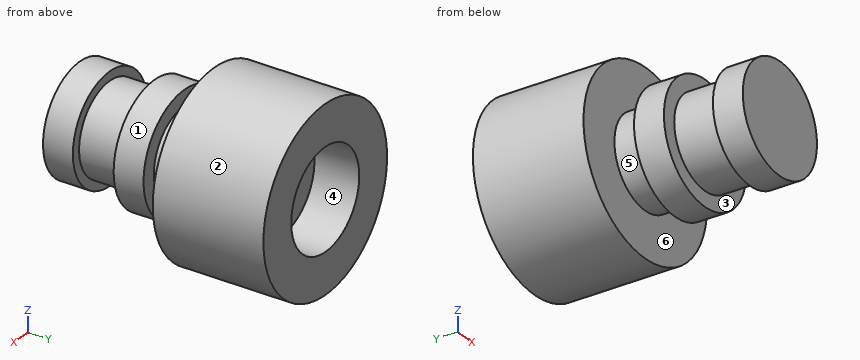
```python
from build123d import *

# Parameters (mm, degrees)
SKETCH1_R           = 3
BOSS_EXTRUDE1_DEPTH = 3.7
SKETCH1_3_R         = 1.6
BOSS_EXTRUDE2_DEPTH = 1
SKETCH5_R           = 1.5
BOSS_EXTRUDE3_DEPTH = 1
SKETCH6_R           = 2
BOSS_EXTRUDE4_DEPTH = 1
SKETCH8_R           = 1.5
BOSS_EXTRUDE5_DEPTH = 2.5
SKETCH10_R          = 1.8
BOSS_EXTRUDE6_DEPTH = 1
SKETCH12_R          = 1.65
CUT_EXTRUDE1_DEPTH  = 1.5


with BuildPart() as part:
    # Sketch1 → Boss-Extrude1 (new body)
    with BuildSketch(Plane(origin=(0, 0, 0), x_dir=(1, 0, 0), z_dir=(0, 1, 0))):
        with Locations((-0.522013312, 0.511138034)):
            Circle(SKETCH1_R)
    extrude(amount=BOSS_EXTRUDE1_DEPTH)

    # Sketch1<3> → Boss-Extrude2 (add)
    with BuildSketch(Plane(origin=(0, 0, 0), x_dir=(1, 0, 0), z_dir=(0, 1, 0))):
        with Locations((-0.522013312, 0.511138034)):
            Circle(SKETCH1_3_R)
    extrude(amount=BOSS_EXTRUDE2_DEPTH)

    # Sketch5 → Boss-Extrude3 (add)
    with BuildSketch(Plane.XZ):
        with Locations((-0.522013312, -0.511138034)):
            Circle(SKETCH5_R)
    extrude(amount=BOSS_EXTRUDE3_DEPTH)

    # Sketch6 → Boss-Extrude4 (add)
    with BuildSketch(Plane.XZ.offset(1)):
        with Locations((-0.522013312, -0.511138034)):
            Circle(SKETCH6_R)
    extrude(amount=BOSS_EXTRUDE4_DEPTH)

    # Sketch8 → Boss-Extrude5 (add)
    with BuildSketch(Plane(origin=(0, -2, 0), x_dir=(-1, 0, 0), z_dir=(0, -1, 0))):
        with Locations((0.522013312, 0.511138034)):
            Circle(SKETCH8_R)
    extrude(amount=BOSS_EXTRUDE5_DEPTH)

    # Sketch10 → Boss-Extrude6 (add)
    with BuildSketch(Plane.XZ.offset(4.5)):
        with Locations((-0.522013312, -0.511138034)):
            Circle(SKETCH10_R)
    extrude(amount=-BOSS_EXTRUDE6_DEPTH)

    # Sketch12 → Cut-Extrude1 (cut)
    with BuildSketch(Plane(origin=(0, 3.7, 0), x_dir=(1, 0, 0), z_dir=(0, 1, 0))):
        with Locations((-0.522013312, 0.511138034)):
            Circle(SKETCH12_R)
    extrude(amount=-CUT_EXTRUDE1_DEPTH, mode=Mode.SUBTRACT)


solid = part.part
```
Geometry: final body of the model. Coordinates: model frame, mm. Face numbers are marked on the shaded views. A direction names the side the tool comes from. Round coordinates to 2 decimals unless told otherwise and drop trailing zeros. Write each loop counter-clockwise with the first axis right and the second up, starting at its lowest first coordinate (ties: lowest second). Pieces come first, ordered by that corner, then holes. Notation, with made-up numbers: M -39.5,66 L 12.5,66 A13 ccw 12.5,89 Z; hole C 42.25,-15.75 d1. An arc over 180 degrees is marked long. Answer in a Markdown table with one row per item. Add a question column.
(1) Draft query along X for the marked faces 4, 5 and 6. Return one class per face: pulls with the +X half, pulls with the -X half, needs draft (parallel to the pull), parting line crosses it, or undercut.
(2) Reachability of the marked faces 1, 2 and 3 from +Z, -Z, +X, -X, +Y, -Y: full face, straight path, thin tool, end or side. Return the list, or none.
(3) Contact query for flat-ended pins moving along their axis: pin 1 (1 mm diameter, centred on x = 0, z = -1, fed in from +Y); pin 2 (1.5 mm diameter, centred on x = -2.5, y = -2.5, fed in from -Z); pin 3 (2 mm diameter, centred on y = 1, z = -2.5, fed in from +X). Output: stop coordinate, or through.
(4) Cut plane D-D, the plane x = -0.95. Return the cut outline in (y, z).
(5) Ray query, L1, parallel to Y at x = 0.4, z = -1.8; L2, parallel to Y at x = -0.3, z = 2; L3, parallel to Z at x = -0.6, y = -3. Return the intervals inside material, ascending.
(6) Cut plane A-A, the plane x = 0.45. Return the cut outline in (y, z).
(7) Cut plane B-B, the plane z = -2.85. Return the cut outline in (x, y), then the cut area to 3 significant figures.
(8) Cut plane C-C, the plane y = 1. Return the cut outline in (x, z), then the cut area to 3 significant figures.
Established:
| question | item | result |
|---|---|---|
| 1 | face 4 | undercut |
| 1 | face 5 | parting line crosses it |
| 1 | face 6 | needs draft |
| 2 | face 1 | -Y |
| 2 | face 2 | +Y, -Y |
| 2 | face 3 | none |
| 3 | pin 1 | y = 2.2 |
| 3 | pin 2 | z = -1.92 |
| 3 | pin 3 | x = 2.31 |
| 4 | outline | M -4.5,-2.26 L -3.5,-2.26 L -3.5,-1.95 L -2,-1.95 L -2,-2.46 L -1,-2.46 L -1,-1.95 L 0,-1.95 L 0,-3.48 L 3.7,-3.48 L 3.7,-2.1 L 2.2,-2.1 L 2.2,1.08 L 3.7,1.08 L 3.7,2.46 L 0,2.46 L 0,0.93 L -1,0.93 L -1,1.44 L -2,1.44 L -2,0.93 L -3.5,0.93 L -3.5,1.24 L -4.5,1.24 Z |
| 5 | L1 | -4.5 to -3.5, -2 to -1, 0 to 2.2 |
| 5 | L2 | 0 to 3.7 |
| 5 | L3 | -2.01 to 0.99 |
| 6 | outline | M -4.5,-2.03 L -3.5,-2.03 L -3.5,-1.65 L -2,-1.65 L -2,-2.26 L -1,-2.26 L -1,-1.65 L 0,-1.65 L 0,-3.35 L 3.7,-3.35 L 3.7,-1.84 L 2.2,-1.84 L 2.2,0.82 L 3.7,0.82 L 3.7,2.33 L 0,2.33 L 0,0.63 L -1,0.63 L -1,1.24 L -2,1.24 L -2,0.63 L -3.5,0.63 L -3.5,1 L -4.5,1 Z |
| 7 | outline | M -2.4,0 L 1.36,0 L 1.36,3.7 L -2.4,3.7 Z |
| 7 | area | 13.9 mm² |
| 8 | outline | C -0.52,-0.51 d6 |
| 8 | area | 28.3 mm² |
